Geometry check sheet. Reference: the model listing, model coordinates, mm. Face numbers are marked on the shaded views. Round coordinates to 2 decimals unless told otherwise and drop trailing zeros. Order: outer loops, then holes, each group sorted by start corner. A loop starts at its lowest first (then second) coordinate and runs counter-clockwise, first axis right, second up.
(1) Cross-section at A-A on x = 0. Enter the section's corners in (y, z).
(2) Thickness scan on L1, parallel to Z at x = 0, y = -11.5; L2, parallel to Z at x = 0, y = 0.65; L3, parallel to Y at x = -2, z = -18. Record the ranges inside material, lowest first.
(3) Gauge pin test, flat ends, axial feed: P1, Ø2, axis at x = 7.5, z = 18, coming from the -Y side; P2, Ø10, axis at y = -17, z = -11, coming from the +X side; P3, Ø5, axis at x = 6, z = 19.5, coming from the -Y side. Record the tip position at first contact, or that the pin passes through.
(4) Cross-section at B-B on z = 0. Enter the section's corners in (x, y), and give its area (3 significant figures).
(5) Draft check along X on the marked faces 1 and 2. Enter one of: pulls with the +X half, pulls with the -X half, needs draft (parallel to the pull), parting line crosses it, or undercut.
(6) Cross-section at C-C on y = -16.75. Enter the section's corners in (x, z), and give its area (3 significant figures).
Autodesk Inventor part; units mm, degrees
ref_plane "YZ Plane" through (0, 0, 0) normal (1, 0, 0) x (0, 1, 0)
ref_plane "XZ Plane" through (0, 0, 0) normal (0, 1, 0) x (-1, 0, 0)
ref_plane "XY Plane" through (0, 0, 0) normal (0, 0, 1) x (1, 0, 0)
sketch "Sketch1" plane through (0, 0, 0) normal (0, 1, 0) x (-1, 0, 0)
  circle A0 centre (0, 0) radius 18
  circle A1 centre (0, 0) radius 25
  dimension "d0" = 36
  dimension "d1" = 50
extrude "Extrusion1" add sketch "Sketch1" along normal blind 2
sketch "Sketch2" plane through (0, 0, 0) normal (0, -1, 0) x (1, 0, 0)
  circle A0 centre (0, 0) radius 25
  circle A1 centre (0, 0) radius 18
  circle A2 centre (0, 0) radius 25
  circle A3 centre (0, 0) radius 24
  dimension "d4" = 48
extrude "Extrusion2" add sketch "Sketch2" along normal blind 10 contours A0
fillet "Fillet1" radius 2 1 edges at (-24, 0, 0)
fillet "Fillet2" radius 2 1 edges at (25, 2, 0)
sketch "Sketch3" plane through (0, -10, 0) normal (0, -1, 0) x (1, 0, 0)
  point P0 (0, 0)
sketch "Sketch4" plane through (0, 2, 0) normal (0, 1, 0) x (1, 0, 0)
  circle A0 centre (0, 0) radius 25
  dimension "d9" = 50
sketch "Sketch5" plane through (0, -10, 0) normal (0, -1, 0) x (1, 0, 0)
  circle A0 centre (0, 0) radius 25
  circle A1 centre (0, 0) radius 24
extrude "Extrusion3" add sketch "Sketch5" along normal blind 10
properties part number "controler_02"
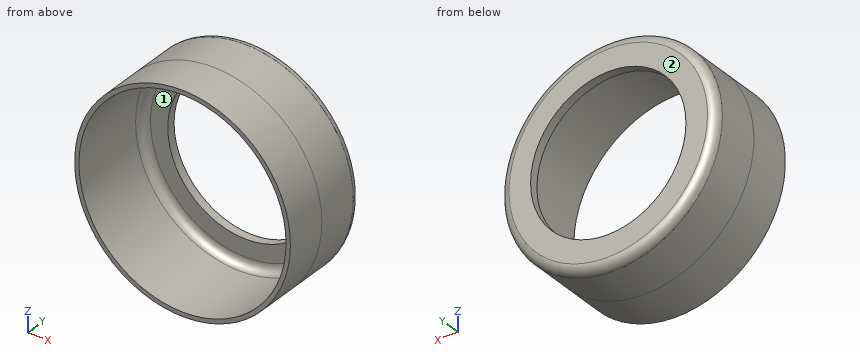
Found:
1. outline: (-20, -25) - (0, -25) arc R2 ccw to (2, -23) - (2, -18) - (0, -18) - (0, -22) arc R2 cw to (-2, -24) - (-20, -24) - close; (-20, 24) - (-2, 24) arc R2 cw to (0, 22) - (0, 18) - (2, 18) - (2, 23) arc R2 ccw to (0, 25) - (-20, 25) - close
2. L1: z = -25 to -24, 24 to 25
2. L2: z = -24.89 to -18, 18 to 24.89
2. L3: y = 0 to 2
3. P1: stops at y = 0
3. P2: stops at x = 24.27
3. P3: stops at y = -0.22
4. outline: (-25, -20) - (-24, -20) - (-24, -2) arc R2 cw to (-22, 0) - (-18, 0) - (-18, 2) - (-23, 2) arc R2 ccw to (-25, 0) - close; (18, 0) - (22, 0) arc R2 cw to (24, -2) - (24, -20) - (25, -20) - (25, 0) arc R2 ccw to (23, 2) - (18, 2) - close
4. area: 68.0 mm2
5. face 1: undercut
5. face 2: needs draft
6. outline: circle Ø50 at (0, 0); hole circle Ø48 at (0, 0)
6. area: 154 mm2
